Model file for the job. Use its own axes, mm. A direction names the side the tool comes from. Round coordinates to 2 decimals unless told otherwise and drop trailing zeros. Order: outer loops, then holes, each group sorted by start corner. A loop starts at its lowest first (then second) coordinate and runs counter-clockwise, first axis right, second up. Notation, with made-up numbers: (70, -34.75) - (117, -34.75) arc R25 cw to (117, -2.75) - close; hole circle Ø7 at (-20.5, 89). An arc over 180 degrees is marked (long way). Write item = value, one per line. Start each with the question number.
from build123d import *

# Parameters (mm, degrees)
ESTRUSIONE_ESTRUSIONE1_DEPTH = 122
SCHIZZO2_W                   = 72
SCHIZZO2_H                   = 55
TAGLIO_ESTRUSIONE1_DEPTH     = 40
SVUOTA1_T                    = -10
SCHIZZO3_R                   = 10
TAGLIO_ESTRUSIONE2_DEPTH     = 40
SCHIZZO4_R                   = 10
TAGLIO_ESTRUSIONE3_DEPTH     = 40
SCHIZZO5_W                   = 152
SCHIZZO5_H                   = 183.793939239
SCHIZZO5_W_2                 = 112
SCHIZZO5_H_2                 = 139.651803616
ESTRUSIONE_ESTRUSIONE2_DEPTH = 5
FORO_PER_VITE_M4_1_D         = 4.5
FORO_PER_VITE_M4_1_DEPTH     = 5
FORO_PER_VITE_M4_1_TIP       = 1.351936393


with BuildPart() as part:
    # Schizzo1 → Estrusione-Estrusione1 (new body)
    with BuildSketch(Plane(origin=(0, 0, 0), x_dir=(0, 0, -1), z_dir=(1, 0, 0))):
        Polygon((0, 0), (0, 35), (-59.39696962, 94.39696962), (-153.793939239, 0), align=None)
    extrude(amount=ESTRUSIONE_ESTRUSIONE1_DEPTH)

    # Schizzo2 → Taglio-Estrusione1 (cut)
    with BuildSketch(Plane(origin=(0, 17.5, -17.5), x_dir=(1, 0, 0), z_dir=(0, 0.7071067811865489, -0.7071067811865461))):
        with Locations((61, -66.748737342)):
            Rectangle(SCHIZZO2_W, SCHIZZO2_H)
    extrude(amount=-TAGLIO_ESTRUSIONE1_DEPTH, mode=Mode.SUBTRACT)

    # Svuota1
    svuota1_openings = [part.faces().sort_by_distance(p)[0] for p in [
        (61, 0, 76.89696962),
    ]]
    offset(amount=SVUOTA1_T, openings=svuota1_openings, kind=Kind.INTERSECTION)

    # Schizzo3 → Taglio-Estrusione2 (cut)
    with BuildSketch(Plane(origin=(0, -10.784271247, 10.784271247), x_dir=(1, 0, 0), z_dir=(0, 0.7071067811865489, -0.7071067811865462))):
        with Locations(Location((61, -66.748737342, 0), (0, 0, 270))):
            Circle(SCHIZZO3_R)
    extrude(amount=-TAGLIO_ESTRUSIONE2_DEPTH, mode=Mode.SUBTRACT)

    # Schizzo4 → Taglio-Estrusione3 (cut)
    with BuildSketch(Plane(origin=(0, 69.825901808, 69.825901808), x_dir=(1, 0, 0), z_dir=(0, -0.7071067811865461, -0.707106781186549))):
        with Locations(Location((61, 73.748737342, 0), (0, 0, 270))):
            Circle(SCHIZZO4_R)
    extrude(amount=-TAGLIO_ESTRUSIONE3_DEPTH, mode=Mode.SUBTRACT)

    # Schizzo5 → Estrusione-Estrusione2 (add)
    with BuildSketch(Plane.XZ):
        with Locations((61, 76.896969619)):
            Rectangle(SCHIZZO5_W, SCHIZZO5_H)
        with Locations((66, 69.825901808)):
            Rectangle(SCHIZZO5_W_2, SCHIZZO5_H_2, mode=Mode.SUBTRACT)
    extrude(amount=-ESTRUSIONE_ESTRUSIONE2_DEPTH)

    # Foro per Vite M4-1
    with Locations(Plane(origin=(0, 5, 0), x_dir=(1, 0, 0), z_dir=(0, 1, 0))):
        with Locations((-7.75, -161.543939239), (129.75, -161.543939239), (129.75, 7.75), (-7.75, 7.75)):
            Hole(FORO_PER_VITE_M4_1_D / 2, depth=FORO_PER_VITE_M4_1_DEPTH)
            with Locations((0, 0, -(FORO_PER_VITE_M4_1_DEPTH + FORO_PER_VITE_M4_1_TIP / 2))):  # 118° drill point
                Cone(0, FORO_PER_VITE_M4_1_D / 2, FORO_PER_VITE_M4_1_TIP, mode=Mode.SUBTRACT)


solid = part.part
Item 1: Which spindle directions (+Z, -Z, +X, -X, +Y, -Y) get a long thin tool onto all of the face, cutting with end or side? Do faces 4 (the face through (60.496, 31.309, 24.197)), 5 (the face through (0, 40, 59)), 6 (the face through (112, 32, 61)), 7 (the face through (52.5, 40.46, 62.03)). Say none if no direction does.
Item 2: Probe L1, parallel to Z at x = -7.75, y = 1.65; L2, parallel to Z at x = 129, y = 1; L3, parallel to Y at x = 94.5, z = 72. List the from-to ranges inside material, lowest first.
Item 3: Saw through at B-B, the plane z = -7.75. Give the cut face in (x, y).
Item 4: Saw through at A-A, the plane x = 129.75. Give the cut face in (y, z), then the cut area to 3 significant figures.
Item 5: Drop flat-ended pins along their axis: pin 1 (7 mm diameter, centred on x = 129.75, z = -7.75, fed in from +Y); pin 2 (6 mm diameter, centred on x = 113.5, y = 61, fed in from -Z); pin 3 (9 mm diameter, centred on x = 68.5, y = 12.5, fed in from -Z); pin 4 (15.5 mm diameter, centred on x = 62, y = 12.5, fed in from +Z). Give the stop position or say it passes through.
Item 6: Saw through at C-C, the plane y = 58.5. Give the cut face in (x, z).
Item 7: Saw through at D-D, the plane x = 46. Give the cut face in (y, z).
Item 8: Mould opens along Z. For faces 1 (the face through (11.65, 55.44, 34.58)), 2 (the face through (60, 20, 0)), 3 (the face through (122, 40, 59)) say: +Z half, -Z half, draft (parallel to the pull), parting line (faces both ways), or undercut.
Check sheet entries:
q1.face_4 = +Y
q1.face_5 = +Z, -Z, -X, +Y
q1.face_6 = -Y
q1.face_7 = none
q2.L1 = -15 to -10, -5.5 to 159.29, 163.79 to 168.79
q2.L2 = -15 to -9.87, -5.63 to 159.42, 163.67 to 168.79
q2.L3 = 36.29 to 50.43, 61.29 to 81.79
q3.outline = (-15, 0) - (-10, 0) - (-10, 5) - (-15, 5) - close; (-5.5, 0) - (127.5, 0) - (127.5, 5) - (-5.5, 5) - close; (132, 0) - (137, 0) - (137, 5) - (132, 5) - close
q4.outline = (0, -15) - (5, -15) - (5, -10) - (0, -10) - close; (0, -5.5) - (5, -5.5) - (5, 159.29) - (0, 159.29) - close; (0, 163.79) - (5, 163.79) - (5, 168.79) - (0, 168.79) - close
q4.area = 874 mm2
q5.pin_1 = 5
q5.pin_2 = 23
q5.pin_3 = 0
q5.pin_4 = 168.79
q6.outline = (0, 23.5) - (25, 23.5) - (25, 74.79) - (97, 74.79) - (97, 23.5) - (122, 23.5) - (122, 95.29) - (0, 95.29) - close; hole (10, 37.64) - (15, 37.64) - (15, 81.15) - (10, 81.15) - close; hole (107, 37.64) - (112, 37.64) - (112, 81.15) - (107, 81.15) - close
q7.outline = (0, -15) - (5, -15) - (5, 0) - (35, 0) - (45.25, 10.25) - (16.97, 38.54) - (55.86, 77.43) - (84.14, 49.14) - (94.4, 59.4) - (5, 148.79) - (5, 168.79) - (0, 168.79) - (0, 139.65) - (51.97, 87.68) - (2.83, 38.54) - (31.11, 10.25) - (30.86, 10) - (0, 10) - close
q8.face_1 = undercut
q8.face_2 = -Z half
q8.face_3 = draft
